from build123d import *

# Parameters (mm, degrees)
SKETCH_1_W          = 300
SKETCH_1_H          = 300
EXTRUDE_1_DEPTH     = 10
SKETCH_2_R          = 20
CUT_EXTRUDE_1_DEPTH = 213.367605816
SKETCH_3_R          = 20
CUT_EXTRUDE_2_DEPTH = 10
SKETCH_4_W          = 35.387588736
SKETCH_4_H          = 35.350682188
CUT_EXTRUDE_3_DEPTH = 25
SKETCH_5_W          = 15.318794368
SKETCH_5_H          = 10
EXTRUDE_2_DEPTH     = 24.5


with BuildPart() as part:
    # 草图1 → 凸台-拉伸1 (new body)
    with BuildSketch(Plane.XY):
        Rectangle(SKETCH_1_W, SKETCH_1_H)
    extrude(amount=EXTRUDE_1_DEPTH)

    # 草图2 → 切除-拉伸1 (cut, through all)
    with BuildSketch(Plane.XY.offset(10)):
        with Locations((35, 20)):
            Circle(SKETCH_2_R)
    extrude(amount=-CUT_EXTRUDE_1_DEPTH, mode=Mode.SUBTRACT)

    # 草图3 → 切除-拉伸2 (cut)
    with BuildSketch(Plane.XY):
        with Locations((80, 80)):
            Circle(SKETCH_3_R)
        with Locations((80, -40)):
            Circle(SKETCH_3_R)
        with Locations((-10, 80)):
            Circle(SKETCH_3_R)
    extrude(amount=CUT_EXTRUDE_2_DEPTH, mode=Mode.SUBTRACT)

    # 草图4 → 切除-拉伸3 (cut)
    with BuildSketch(Plane.XY.offset(10)):
        with Locations((-152.375, -137.625)):
            Rectangle(SKETCH_4_W, SKETCH_4_H)
    extrude(amount=-CUT_EXTRUDE_3_DEPTH, mode=Mode.SUBTRACT)

    # 草图5 → 凸台-拉伸2 (add)
    with BuildSketch(Plane.XZ.offset(119.949658906)):
        with Locations((-142.340602816, 5)):
            Rectangle(SKETCH_5_W, SKETCH_5_H)
    extrude(amount=EXTRUDE_2_DEPTH)


solid = part.part
The listing builds one solid part. Answer for the finished solid, in the listing's coordinates (mm). A direction names the side the tool comes from. Coordinates: 2 decimals unless noted, no trailing zeros. Loops run counter-clockwise (first coordinate to the right, second up) from the corner with the lowest first, then second, coordinate; pieces in that order, holes last.
1) Find section A-A on x = 35. Write down the section's boundary in (y, z).
2) A tool of negligible diameter and unlimited length cuts with its end or side. For faces 4 (the face through (-142, -144.45, 5)), 5 (the face through (75.664, 60.476, 4.93)), from which of +Z, -Z, +X, -X, +Y, -Y can it reach the whole face along a straight path? Write none if from no direction.
3) Find section B-B on y = -40. Write down the section's boundary in (x, z).
4) Find the intervals of material crossed by L1, parallel to Y at x = 80, z = 6.25; L2, parallel to Y at x = 84, z = 9.25; L3, parallel to Y at x = 35, z = 4.5, in increasing order.
5) A flat-ended cylindrical pin translates along its axis: pin 1 Ø4.5 at (y, z) = (-147, 3.5) entering from -X. Find the tip coordinate at first contact, or state that the pin passes through.
6) Find section C-C on z = 5.75. Write down the section's boundary in (x, y).
7) Determine the mould class of faces 1 (the face through (-2, 150, 5)), 2 (the face through (77.4, -20.17, 4.93)), 3 (the face through (6, -150, 5)) for opening direction Y: pulls with the +Y half, pulls with the -Y half, needs draft (parallel to the pull), parting line crosses it, or undercut.
8) Find section D-D on x = 80. Write down the section's boundary in (y, z), then the cut area to 3 significant figures.
Values:
1. outline: (-150, 0) - (0, 0) - (0, 10) - (-150, 10) - close; (40, 0) - (150, 0) - (150, 10) - (40, 10) - close
2. face 4: +Z, -Z, -X, -Y
2. face 5: +Z, -Z
3. outline: (-150, 0) - (60, 0) - (60, 10) - (-150, 10) - close; (100, 0) - (150, 0) - (150, 10) - (100, 10) - close
4. L1: y = -150 to -60, -20 to 60, 100 to 150
4. L2: y = -150 to -59.6, -20.4 to 60.4, 99.6 to 150
4. L3: y = -150 to 0, 40 to 150
5. pin 1: stops at x = -134.68
6. outline: (-150, -144.45) - (-134.68, -144.45) - (-134.68, -150) - (150, -150) - (150, 150) - (-150, 150) - close; hole circle Ø40 at (-10, 80); hole circle Ø40 at (35, 20); hole circle Ø40 at (80, -40); hole circle Ø40 at (80, 80)
7. face 1: pulls with the +Y half
7. face 2: undercut
7. face 3: pulls with the -Y half
8. outline: (-150, 0) - (-60, 0) - (-60, 10) - (-150, 10) - close; (-20, 0) - (60, 0) - (60, 10) - (-20, 10) - close; (100, 0) - (150, 0) - (150, 10) - (100, 10) - close
8. area: 2,200 mm2
